Check sheet for the modelled part. Datum: model origin and axes. Units: mm. Give positions to 0.01 mm unless a question says otherwise; leave off trailing zeros. Write each loop counter-clockwise with the first axis right and the second up, starting at its lowest first coordinate (ties: lowest second). Pieces come first, ordered by that corner, then holes. Notation, with made-up numbers: (78.5, 75) -> (93.5, 75) arc R30 ccw to (93.5, 103) -> close; hole circle Ø4 at (-39, 81.5). An arc over 180 degrees is marked (long way). Answer as a JSON object with one key per item and string values.
from build123d import *

# Parameters (mm, degrees)
REVOLVE1_ANGLE = 280
FILLET1_DEPTH  = 4
FILLET2_R      = 1.2


with BuildPart() as part:
    # Sketch1 → Revolve1 (revolve)
    with BuildSketch(Plane.XY):
        Polygon((13, 0), (13, 0.8), (15, 2.8), (16, 2.8), (16, 0), align=None)
    revolve(axis=Axis((0, 0, 0), (0, 1, 0)), revolution_arc=REVOLVE1_ANGLE)

    # Fillet1: read off the stored shape, not the designer's step
    # Fillet1 outline → Fillet1 (cut)
    with BuildSketch(Plane(origin=(0, 0, 0), x_dir=(1, 0, 0), z_dir=(0, 1, 0))):
        with BuildLine():
            Line((13, 0), (16, 0))
            ThreePointArc((16, 0), (13.674960129, 2.07014875), (12.099184783, 4.754968727))
            ThreePointArc((12.099184783, 4.754968727), (12.77281101, 2.419772492), (13, 0))
        make_face()
        with BuildLine():
            ThreePointArc((2.25742631, -12.802500789), (-0.165035355, -12.998952394), (-2.581728679, -12.741062633))
            ThreePointArc((-2.581728679, -12.741062633), (0.335933367, -13.826684315), (2.778370843, -15.756924048))
            Line((2.778370843, -15.756924048), (2.25742631, -12.802500789))
        make_face()
    extrude(amount=FILLET1_DEPTH, mode=Mode.SUBTRACT)

    # Fillet2
    fillet2_edges = [part.edges().sort_by_distance(p)[0] for p in [
        (16, 1.4, 0),
        (2.778370843, 1.4, 15.756924048),
    ]]
    fillet(fillet2_edges, radius=FILLET2_R)


solid = part.part
1. Go/stop test with flat-tipped pins: P1, Ø1, axis at x = -9, y = 0.5, coming from the -Z side; P2, Ø12, axis at x = -10.5, z = -5, coming from the +Y side; P3, Ø5, axis at x = -6.5, z = -7, coming from the +Y side; P4, Ø2, axis at x = -2.5, z = 12, coming from the +Y side. Record where each tip stops, or that it passes through.
Determined:
{"P1": "z = -13.56", "P2": "y = 2.8", "P3": "through", "P4": "y = 1.06"}
2. Mould release check, pull along Z, two halves, no side actions. Record for faces 1 (the face through (-11.93, 1.38, -10.66)), 2 (the face through (-11, 2.8, -11)), 3 (the face through (-0.88, 0.588, 13.247)), 4 (the face through (12.914, 0.588, -3.132)): released by +Z, released by -Z, zero draft, split by the parting line, or undercut.
Determined:
{"face 1": "split by the parting line", "face 2": "zero draft", "face 3": "undercut", "face 4": "released by +Z"}
3. Sectioned sample at A-A, the plane z = 0. Enter the section's corners in (x, y), plus the area to 3 significant figures.
Determined:
{"outline": "(-16, 0) -> (-13, 0) -> (-13, 0.8) -> (-15, 2.8) -> (-16, 2.8) -> close", "area": "6.40 mm^2"}
4. Scan lines: L1, parallel to X at y = 0.5, z = 0; L2, parallel to Z at x = -1.5, y = 1.5; L3, parallel to Z at x = 0, y = 0.3. Record each from-to range of solid material in increasing order. Write a range as [from, to].
Determined:
{"L1": "[-16, -13]", "L2": "[-15.93, -13.62], [13.62, 15.93]", "L3": "[-16, -13], [13.65, 15.93]"}
